Here's how the part is built. I have some questions about the finished solid (model axes, mm). Give positions to 0.01 mm unless a question says otherwise; leave off trailing zeros. Order: outer loops, then holes, each group sorted by start corner. A loop starts at its lowest first (then second) coordinate and runs counter-clockwise, first axis right, second up.
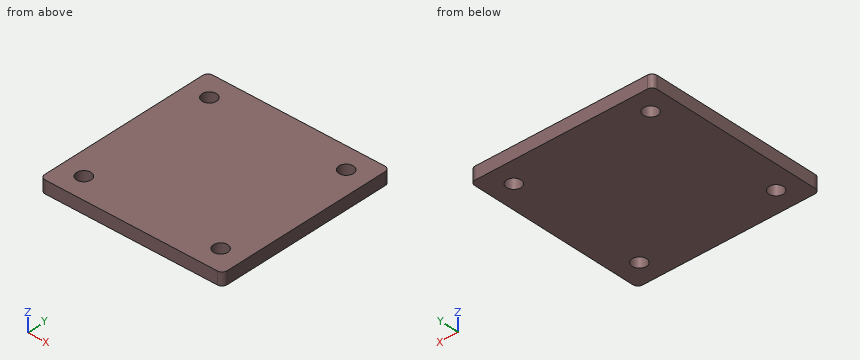
from build123d import *

# Parameters (mm, degrees)
SKETCH1_W           = 72
SKETCH1_H           = 72
SKETCH1_R           = 2.85
BOSS_EXTRUDE1_DEPTH = 5
FILLET1_R           = 2
FILLET2_R           = 2


with BuildPart() as part:
    # Sketch1 → Boss-Extrude1 (new body)
    with BuildSketch(Plane.XY):
        Rectangle(SKETCH1_W, SKETCH1_H)
        with Locations((-27, 27)):
            Circle(SKETCH1_R, mode=Mode.SUBTRACT)
        with Locations((27, 27)):
            Circle(SKETCH1_R, mode=Mode.SUBTRACT)
        with Locations((27, -27)):
            Circle(SKETCH1_R, mode=Mode.SUBTRACT)
        with Locations((-27, -27)):
            Circle(SKETCH1_R, mode=Mode.SUBTRACT)
    extrude(amount=BOSS_EXTRUDE1_DEPTH)

    # Fillet1
    fillet1_edges = [part.edges().sort_by_distance(p)[0] for p in [
        (-36, 36, 2.5),
    ]]
    fillet(fillet1_edges, radius=FILLET1_R)

    # Fillet2
    fillet2_edges = [part.edges().sort_by_distance(p)[0] for p in [
        (36, 36, 2.5),
        (36, -36, 2.5),
        (-36, -36, 2.5),
    ]]
    fillet(fillet2_edges, radius=FILLET2_R)


solid = part.part
Q1. I need wall thicknesses on L1, parallel to Y at x = -27, z = 3.1; L2, parallel to Y at x = -28, z = 4.3. Which ranges of each line are inside material? Lowest first, please.
Filled sheet:
L1: y = -36 to -29.85, -24.15 to 24.15, 29.85 to 36
L2: y = -36 to -29.67, -24.33 to 24.33, 29.67 to 36
Q2. If we section it at B-B on z = 3.1: List the corners of the cut face in (x, y) for me.
Filled sheet:
outline: (-36, -34) arc R2 ccw to (-34, -36) - (34, -36) arc R2 ccw to (36, -34) - (36, 34) arc R2 ccw to (34, 36) - (-34, 36) arc R2 ccw to (-36, 34) - close; hole circle Ø5.7 at (-27, -27); hole circle Ø5.7 at (-27, 27); hole circle Ø5.7 at (27, -27); hole circle Ø5.7 at (27, 27)
Q3. If we section it at A-A on x = 27: List the corners of the cut face in (y, z) for me, plus the area to 3 significant figures.
Filled sheet:
outline: (-36, 0) - (-29.85, 0) - (-29.85, 5) - (-36, 5) - close; (-24.15, 0) - (24.15, 0) - (24.15, 5) - (-24.15, 5) - close; (29.85, 0) - (36, 0) - (36, 5) - (29.85, 5) - close
area: 303 mm2
Q4. I'm going to push a flat-ended pin straight in: P1, Ø5, axis at x = -27, y = -27, coming from the +Z side. Where does the tip first touch, or does it pass through?
Filled sheet:
P1: passes through
